from build123d import *

# Parameters (mm, degrees)
SKETCH1_R           = 1.5
BOSS_EXTRUDE1_DEPTH = 4
SKETCH2_W           = 20
SKETCH2_H           = 0.5
CUT_EXTRUDE1_DEPTH  = 15.044571905
FILLET1_R           = 0.5
FILLET2_R           = 0.75


with BuildPart() as part:
    # Sketch1 → Boss-Extrude1 (new body)
    with BuildSketch(Plane(origin=(0, 0, 0), x_dir=(1, 0, 0), z_dir=(0, 1, 0))):
        with BuildLine():
            Line((-2.5, -10), (-2.5, 10))
            ThreePointArc((-2.5, 10), (0, 12.5), (2.5, 10))
            Line((2.5, 10), (2.5, -10))
            ThreePointArc((2.5, -10), (0, -12.5), (-2.5, -10))
        make_face()
        with Locations(Location((0, -10, 0), (0, 0, 270))):
            Circle(SKETCH1_R, mode=Mode.SUBTRACT)
        with Locations(Location((0, 10, 0), (0, 0, 270))):
            Circle(SKETCH1_R, mode=Mode.SUBTRACT)
    extrude(amount=BOSS_EXTRUDE1_DEPTH)

    # Sketch2 → Cut-Extrude1 (cut, through all)
    with BuildSketch(Plane(origin=(2.5, 0, 0), x_dir=(0, 0, -1), z_dir=(1, 0, 0))):
        with Locations((0, 0.25)):
            Rectangle(SKETCH2_W, SKETCH2_H)
    extrude(amount=-CUT_EXTRUDE1_DEPTH, mode=Mode.SUBTRACT)

    # Fillet1
    fillet1_edges = [part.edges().sort_by_distance(p)[0] for p in [
        (2.5, 0.5, 0),
        (-2.5, 0.5, 0),
    ]]
    fillet(fillet1_edges, radius=FILLET1_R)

    # Fillet2
    # the kernel refuses this fillet: 0.75 mm, written as the material it takes off along each edge
    with BuildSketch(Plane(origin=(0, 4, 10), x_dir=(0, 0, 1), z_dir=(-1, 0, 0))) as fillet2_piece_1:
        with BuildLine():
            CenterArc((1.5 + FILLET2_R, -FILLET2_R), FILLET2_R, 90, 90)
            Line((1.5 + FILLET2_R, 0), (1.5, 0))
            Line((1.5, 0), (1.5, -FILLET2_R))
        make_face()
    revolve(axis=Axis((0, 4, 10), (0, 1, 0)), mode=Mode.SUBTRACT)
    with BuildSketch(Plane(origin=(0, 4, -10), x_dir=(-1, 0, 0), z_dir=(0, 0, 1))) as fillet2_piece_2:
        with BuildLine():
            CenterArc((2.5 - FILLET2_R, FILLET2_R), FILLET2_R, 270, 90)
            Line((2.5 - FILLET2_R, 0), (2.5, 0))
            Line((2.5, 0), (2.5, FILLET2_R))
        make_face()
    revolve(axis=Axis((0, 4, -10), (0, -1, 0)), revolution_arc=180, mode=Mode.SUBTRACT)
    with BuildSketch(Plane(origin=(0, 4, -10), x_dir=(0, 0, 1), z_dir=(-1, 0, 0))) as fillet2_piece_3:
        with BuildLine():
            CenterArc((1.5 + FILLET2_R, -FILLET2_R), FILLET2_R, 90, 90)
            Line((1.5 + FILLET2_R, 0), (1.5, 0))
            Line((1.5, 0), (1.5, -FILLET2_R))
        make_face()
    revolve(axis=Axis((0, 4, -10), (0, 1, 0)), mode=Mode.SUBTRACT)
    with BuildSketch(Plane(origin=(-2.5, 4, 10), x_dir=(1, 0, 0), z_dir=(0, 0, -1))) as fillet2_piece_4:
        with BuildLine():
            CenterArc((FILLET2_R, FILLET2_R), FILLET2_R, 180, 90)
            Line((0, FILLET2_R), (0, 0))
            Line((0, 0), (FILLET2_R, 0))
        make_face()
    extrude(amount=20, mode=Mode.SUBTRACT)
    with BuildSketch(Plane(origin=(0, 4, 10), x_dir=(1, 0, 0), z_dir=(0, 0, -1))) as fillet2_piece_5:
        with BuildLine():
            CenterArc((2.5 - FILLET2_R, FILLET2_R), FILLET2_R, 270, 90)
            Line((2.5 - FILLET2_R, 0), (2.5, 0))
            Line((2.5, 0), (2.5, FILLET2_R))
        make_face()
    revolve(axis=Axis((0, 4, 10), (0, -1, 0)), revolution_arc=180, mode=Mode.SUBTRACT)
    with BuildSketch(Plane(origin=(2.5, 4, -10), x_dir=(0, -1, 0), z_dir=(0, 0, 1))) as fillet2_piece_6:
        with BuildLine():
            CenterArc((FILLET2_R, -FILLET2_R), FILLET2_R, 90, 90)
            Line((0, -FILLET2_R), (0, 0))
            Line((0, 0), (FILLET2_R, 0))
        make_face()
    extrude(amount=20, mode=Mode.SUBTRACT)


solid = part.part
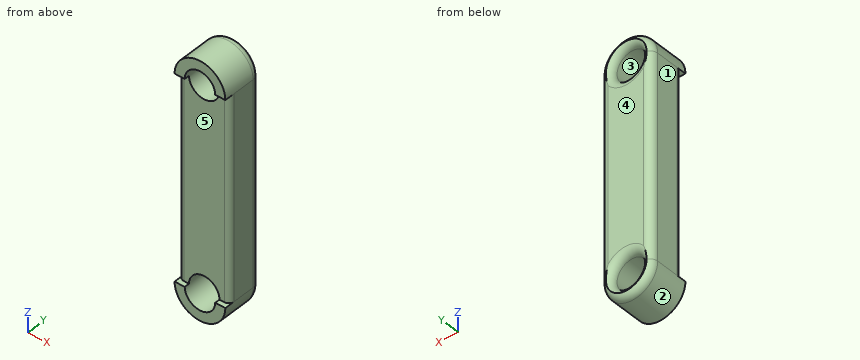
Read the model definition and answer for the solid it produces. Units are mm, in the model's axes. Face numbers are marked on the shaded views. A direction names the side the tool comes from. Coordinates: 2 decimals unless noted, no trailing zeros. Loops run counter-clockwise (first coordinate to the right, second up) from the corner with the lowest first, then second, coordinate; pieces in that order, holes last. Notation, with made-up numbers: (33, -18.75) - (77, -18.75) arc R26 ccw to (77, 5.25) - close; hole circle Ø4 at (-1, 15). An arc over 180 degrees is marked (long way). Answer in a Markdown table with one row per item.
Q1. Straight lines are drawn through the part: line 1 along Z through (x, y) = (0, 0.75); line 2 along X through (y, z) = (2.45, 10); line 3 along Z through (x, y) = (1.35, 2.35). For each, find the intervals that lie inside material, in ascending order. Write a range as [from, to].
Here are the results:
| item | result |
|---|---|
| line 1 | z = [-12.5, -11.5], [-8.5, 8.5], [11.5, 12.5] |
| line 2 | x = [-2.5, -1.5], [1.5, 2.5] |
| line 3 | z = [-12.1, -10.65], [-9.35, 9.35], [10.65, 12.1] |
Q2. For the marked faces 4 and 5, determine the directions among +Z, -Z, +X, -X, +Y, -Y from which every point of the face is accessible in a straight line to the end or side of a thin tool.
Here are the results:
| item | result |
|---|---|
| face 4 | +Z, -Z, +X, -X, +Y |
| face 5 | +X, -X, -Y |
Q3. Find section A-A on x = 0. Write down the section's boundary in (y, z).
Here are the results:
| item | result |
|---|---|
| outline | (0, -12.5) - (3.25, -12.5) arc R0.75 ccw to (3.96, -12) arc R0.75 ccw to (3.25, -11.5) - (0, -11.5) - close; (0, 11.5) - (3.25, 11.5) arc R0.75 ccw to (3.96, 12) arc R0.75 ccw to (3.25, 12.5) - (0, 12.5) - close; (0.5, -8.5) - (3.25, -8.5) arc R0.75 ccw to (4, -7.75) - (4, 7.75) arc R0.75 ccw to (3.25, 8.5) - (0.5, 8.5) - close |
Q4. Find section D-D on x = -1.15. Count the separate pieces of the cut face and the enclosed holes in it, plus the area to 3 significant figures.
Here are the results:
| item | result |
|---|---|
| separate pieces | 3 |
| enclosed holes | 0 |
| area | 72.4 mm^2 |
Q5. Find section B-B on y = 2.95. Write down the section's boundary in (x, z), plus the area to 3 significant figures.
Here are the results:
| item | result |
|---|---|
| outline | (-2.5, -10) arc R2.5 ccw to (2.5, -10) - (2.5, 10) arc R2.5 ccw to (-2.5, 10) - close; hole circle Ø3 at (0, -10); hole circle Ø3 at (0, 10) |
| area | 105 mm^2 |
Q6. The mould has two halves that part along Z. Classify the marked faces 1, 2 and 3: pulls with the +Z half, pulls with the -Z half, needs draft (parallel to the pull), parting line crosses it, or undercut.
Here are the results:
| item | result |
|---|---|
| face 1 | needs draft |
| face 2 | pulls with the -Z half |
| face 3 | undercut |
Q7. Find section C-C on z = 1.75. Write down the section's boundary in (x, y), plus the area to 3 significant figures.
Here are the results:
| item | result |
|---|---|
| outline | (-2.5, 1) arc R0.5 ccw to (-2, 0.5) - (2, 0.5) arc R0.5 ccw to (2.5, 1) - (2.5, 3.25) arc R0.75 ccw to (1.75, 4) - (-1.75, 4) arc R0.75 ccw to (-2.5, 3.25) - close |
| area | 17.2 mm^2 |
Q8. Given P1, Ø0.5, axis at x = -2, y = 0.5, coming from the -Z side; P2, Ø1.2, axis at x = -0.5, z = 4, coming from the -Y side; P3, Ø0.5, axis at x = 2, y = 0.5, coming from the +Z side; P4, Ø2.5, axis at x = 0, z = -10, coming from the -Y side, each flat-ended and moving along its own axis, determine where each tip first touches the part or whether it passes through.
Here are the results:
| item | result |
|---|---|
| P1 | stops at z = -11.79 |
| P2 | stops at y = 0.5 |
| P3 | stops at z = 11.79 |
| P4 | passes through |
